Drawing for the job (mm, zero at the part's lowest x, y, z). A direction names the side the tool comes from. Coordinates: 2 decimals unless noted, no trailing zeros. Order: outer loops, then holes, each group sorted by start corner. A loop starts at its lowest first (then second) coordinate and runs counter-clockwise, first axis right, second up.
1) Mould opens along X. For the marked faces 1, 2 and 3 say: +X half, -X half, draft (parallel to the pull), parting line (faces both ways), or undercut.
2) Cut at A-A (z = 4.75). List the corners of the cut face in (x, y), and give its area (3 significant figures).
3) Cut at C-C (x = 4.5). List the corners of the cut face in (y, z).
4) Pin check, flat tips, straight feed: pin 1 Ø2 at (x, y) = (2.5, 13.5) entering from -Z; pin 2 Ø3 at (x, y) = (1.5, 6.5) entering from +Z; pin 3 Ø2 at (y, z) = (13, 5) entering from -X. Stop position of each tip, or through.
5) Cut at D-D (x = 8). List the corners of the cut face in (y, z).
6) Wall check: L1, parallel to Y at x = 4.5, z = 7.2; L2, parallel to Y at x = 7.25, z = 3.75; L3, parallel to X at y = 10, z = 7.7. Give the ranges that are in metal, low to high.
7) Cut at B-B (y = 10). List the corners of the cut face in (x, z).
8) Tool access for the marked faces 4, 5 and 6: list every direction of +Z, -Z, +X, -X, +Y, -Y with a clear straight run to the whole face (end or side of a thin tool).
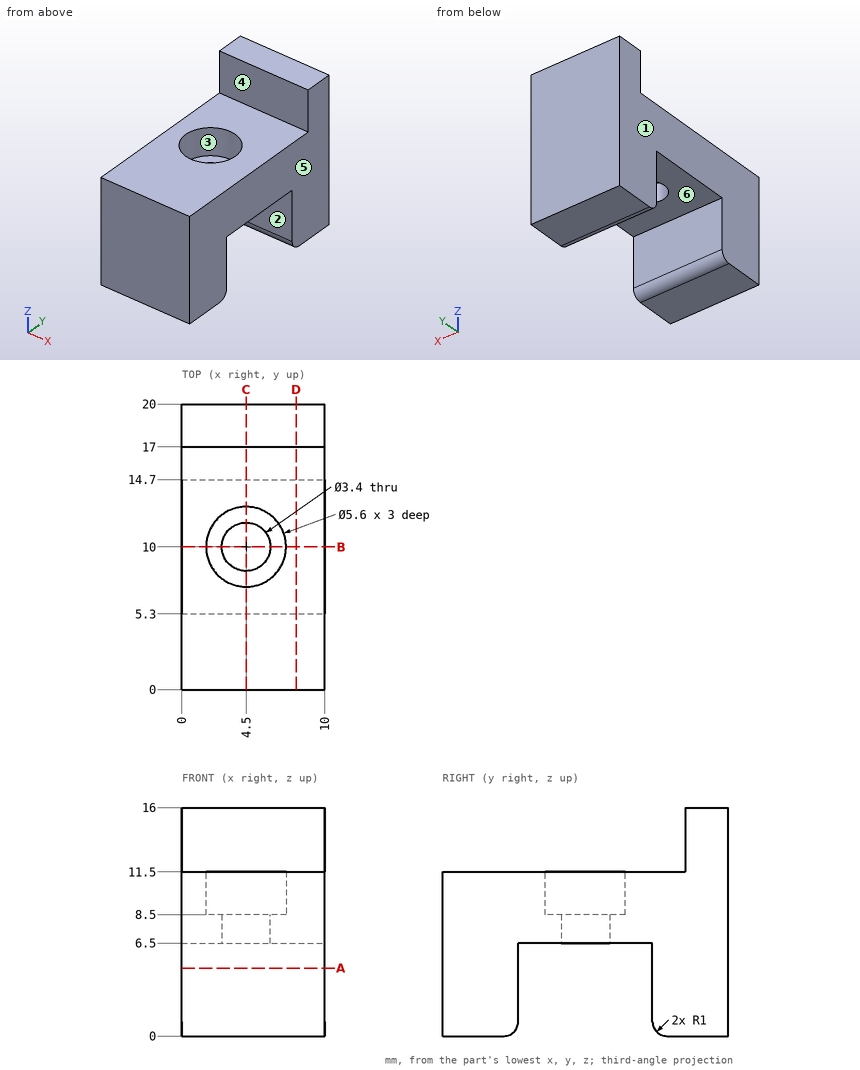
Geometry check:
1. face 1: -X half
1. face 2: draft
1. face 3: undercut
2. outline: (0, 0) - (10, 0) - (10, 5.3) - (0, 5.3) - close; (0, 14.7) - (10, 14.7) - (10, 20) - (0, 20) - close
2. area: 106 mm2
3. outline: (0, 0) - (4.3, 0) arc R1 ccw to (5.3, 1) - (5.3, 6.5) - (8.3, 6.5) - (8.3, 8.5) - (7.2, 8.5) - (7.2, 11.5) - (0, 11.5) - close; (11.7, 6.5) - (14.7, 6.5) - (14.7, 1) arc R1 ccw to (15.7, 0) - (20, 0) - (20, 16) - (17, 16) - (17, 11.5) - (12.8, 11.5) - (12.8, 8.5) - (11.7, 8.5) - close
4. pin 1: stops at z = 6.5
4. pin 2: stops at z = 11.5
4. pin 3: passes through
5. outline: (0, 0) - (4.3, 0) arc R1 ccw to (5.3, 1) - (5.3, 6.5) - (14.7, 6.5) - (14.7, 1) arc R1 ccw to (15.7, 0) - (20, 0) - (20, 16) - (17, 16) - (17, 11.5) - (0, 11.5) - close
6. L1: y = 0 to 8.3, 11.7 to 20
6. L2: y = 0 to 5.3, 14.7 to 20
6. L3: x = 0 to 2.8, 6.2 to 10
7. outline: (0, 6.5) - (2.8, 6.5) - (2.8, 8.5) - (1.7, 8.5) - (1.7, 11.5) - (0, 11.5) - close; (6.2, 6.5) - (10, 6.5) - (10, 11.5) - (7.3, 11.5) - (7.3, 8.5) - (6.2, 8.5) - close
8. face 4: +Z, +X, -X, -Y
8. face 5: +Z, -Z, +X, +Y, -Y
8. face 6: -Z, +X, -X
